Geometry check sheet. Reference: the model listing, model coordinates, mm. A direction names the side the tool comes from. Coordinates: 2 decimals unless noted, no trailing zeros. Loops run counter-clockwise (first coordinate to the right, second up) from the corner with the lowest first, then second, coordinate; pieces in that order, holes last.
from build123d import *

# Parameters (mm, degrees)
BOSS_EXTRUDE1_DEPTH = 50.8
SKETCH2_W           = 41.275
SKETCH2_H           = 19.05
SKETCH2_W_2         = 88.9
SKETCH2_H_2         = 22.225
CUT_EXTRUDE2_DEPTH  = 48.625
SKETCH3_R           = 6.35
BOSS_EXTRUDE2_DEPTH = 3.175
SKETCH4_W           = 88.9
SKETCH4_H           = 9.525
BOSS_EXTRUDE3_DEPTH = 22.225
SKETCH5_W           = 28.575
SKETCH5_H           = 4.7625
BOSS_EXTRUDE4_DEPTH = 4.7625
FILLET1_R           = 6.35
SKETCH6_R           = 6.35
CUT_EXTRUDE3_DEPTH  = 29.5750001


with BuildPart() as part:
    # Sketch1 → Boss-Extrude1 (new body)
    with BuildSketch(Plane.XY):
        with BuildLine():
            Line((-14.2875, 47.625), (-74.6125, 47.625))
            Line((-74.6125, 47.625), (-74.6125, 19.05))
            ThreePointArc((-74.6125, 19.05), (-77.402307909, 12.314807909), (-84.1375, 9.525))
            Line((-84.1375, 9.525), (-88.9, 9.525))
            Line((-88.9, 9.525), (-88.9, 0))
            Line((-88.9, 0), (0, 0))
            Line((0, 0), (0, 9.525))
            Line((0, 9.525), (-4.7625, 9.525))
            ThreePointArc((-4.7625, 9.525), (-11.497692091, 12.314807909), (-14.2875, 19.05))
            Line((-14.2875, 19.05), (-14.2875, 47.625))
        make_face()
    extrude(amount=BOSS_EXTRUDE1_DEPTH)

    # Sketch2 → Cut-Extrude2 (cut, through all)
    with BuildSketch(Plane(origin=(0, 47.625, 0), x_dir=(1, 0, 0), z_dir=(0, 1, 0))):
        with Locations((-44.45, -9.525)):
            Rectangle(SKETCH2_W, SKETCH2_H)
        with Locations((-44.45, -39.6875)):
            Rectangle(SKETCH2_W_2, SKETCH2_H_2)
    extrude(amount=-CUT_EXTRUDE2_DEPTH, mode=Mode.SUBTRACT)

    # Sketch3 → Boss-Extrude2 (add)
    with BuildSketch(Plane.XY.offset(28.575)):
        with BuildLine():
            Line((-58.7375, 28.575), (-58.7375, 9.525))
            Line((-58.7375, 9.525), (-30.1625, 9.525))
            Line((-30.1625, 9.525), (-30.1625, 28.575))
            ThreePointArc((-30.1625, 28.575), (-44.45, 42.8625), (-58.7375, 28.575))
        make_face()
        with Locations((-44.45, 28.575)):
            Circle(SKETCH3_R, mode=Mode.SUBTRACT)
    extrude(amount=BOSS_EXTRUDE2_DEPTH)

    # Sketch4 → Boss-Extrude3 (add)
    with BuildSketch(Plane.XY.offset(28.575)):
        with Locations((-44.45, 4.7625)):
            Rectangle(SKETCH4_W, SKETCH4_H)
    extrude(amount=BOSS_EXTRUDE3_DEPTH)

    # Sketch5 → Boss-Extrude4 (add)
    with BuildSketch(Plane.XY.offset(31.75)):
        with Locations((-44.45, 11.90625)):
            Rectangle(SKETCH5_W, SKETCH5_H)
    extrude(amount=BOSS_EXTRUDE4_DEPTH)

    # Fillet1
    fillet1_edges = [part.edges().sort_by_distance(p)[0] for p in [
        (-88.9, 4.7625, 0),
        (-88.9, 4.7625, 50.8),
        (0, 4.7625, 50.8),
        (0, 4.7625, 0),
    ]]
    fillet(fillet1_edges, radius=FILLET1_R)

    # Sketch6 → Cut-Extrude3 (cut, through all)
    with BuildSketch(Plane.XY.offset(28.575)):
        with Locations((-44.45, 28.575)):
            Circle(SKETCH6_R)
    extrude(amount=-CUT_EXTRUDE3_DEPTH, mode=Mode.SUBTRACT)


solid = part.part
(1) Sectioned sample at D-D on z = 42.5. Record the cut outline in (x, y) (3 decimals), and give its area (3 significant figures).
Findings:
outline: (-88.9, 0) - (0, 0) - (0, 9.525) - (-88.9, 9.525) - close
area: 847 mm2
(2) Access from +Z, -Z, +X, -X, +Y, -Y to the whole of each face (thin tool, end or side, straight path). Record for faces 5 (the flat face through (-54, 42, 28.575)), 6 (the flat face through (-30.162, 17, 31)), 7 (the flat face through (-45, 14.288, 34)), 8 (the flat face through (-14.288, 33, 14)), 9 (the flat face through (-49.3, 24.1, 19.05)).
Findings:
face 5: +Z, +Y
face 6: +Z, +X, +Y
face 7: +Z, +X, -X, +Y
face 8: +Z, -Z, +X, +Y
face 9: -Z, +Y, -Y
(3) Gauge pin test, flat ends, axial feed: pin 1 Ø5.5 at (y, z) = (13, 9) entering from -X; pin 2 Ø5 at (x, y) = (-27.5, 30.5) entering from -Z; pin 3 Ø6 at (y, z) = (35, 30) entering from +X; pin 4 Ø11.5 at (x, y) = (-44.45, 28.575) entering from +Z. Record the tip position at first contact, or that the pin passes through.
Findings:
pin 1: stops at x = -80.49
pin 2: stops at z = 19.05
pin 3: stops at x = -14.29
pin 4: passes through
(4) Scan lines: L1, parallel to Y at x = -44, z = 24 (3 decimals); L2, parallel to X at y = 29, z = 22; L3, parallel to X at y = 29, z = 18.5. Record each from-to range of solid material in increasing order.
Findings:
L1: y = 0 to 22.241, 34.909 to 47.625
L2: x = -74.61 to -50.79, -38.11 to -14.29
L3: x = -74.61 to -65.09, -23.81 to -14.29
(5) Draft check along X on faces 1 (the cylindrical face through (-44.14, 42.86, 30.14)), 2 (the flat face through (-65.088, 24, 10)), 3 (the flat face through (-23.813, 24, 10)), 4 (the flat face through (-72, 19, 0)). Enter one of: +X half, -X half, draft (parallel to the pull), parting line (faces both ways), or undercut.
Findings:
face 1: parting line
face 2: undercut
face 3: undercut
face 4: draft
